from build123d import *

# Parameters (mm, degrees)
F0_W     = 18
F0_H     = 18
F1_DEPTH = 9


with BuildPart() as f1:
    # F0 (on Front) → F1 (new body, symmetric)
    with BuildSketch(Plane.XZ):
        Rectangle(F0_W, F0_H)
    extrude(amount=F1_DEPTH, both=True)


with BuildPart() as f3:
    # F2 (on Front) → F3 (revolve)
    with BuildSketch(Plane.XZ):
        with BuildLine():
            Line((-12.727922, 0), (12.727922, 0))
            ThreePointArc((12.727922, 0), (0, 12.727922), (-12.727922, 0))
        make_face()
    revolve(axis=Axis((0.310661, 0, 0), (1, 0, 0)))


with BuildPart() as f1_1:
    add(f1.part)

    # F4: intersect F3
    add(f3.part, mode=Mode.INTERSECT)


solid = f1_1.part
For this review, take the finished solid that the model builds, in its own axes (mm). Round coordinates to 2 decimals unless told otherwise and drop trailing zeros. Order: outer loops, then holes, each group sorted by start corner. A loop starts at its lowest first (then second) coordinate and runs counter-clockwise, first axis right, second up. Notation, with made-up numbers: (46, -4.5) -> (60, -4.5) arc R20 ccw to (60, 20.5) -> close; hole circle Ø4 at (43.5, -37.75). An arc over 180 degrees is marked (long way). Write item = value, one per line. Start each with the question number.
1) Take a section at B-B on y = 8. State the section outline as (x, z) points, plus the area to 3 significant figures.
2) Take a section at A-A on z = 8.25. State the section outline as (x, y) points.
3) To check wall thickness, follow line 1 (X direction, y = 7.25, z = -6.5); line 2 (X direction, y = -7.75, z = 8.25); line 3 (Z direction, x = 5.25, y = 7.75). State the ranges of each line that lie inside material, in increasing order. Write a range as from..to.
Verdict:
q1.outline = (-9, -4.12) arc R9.9 ccw to (-4.12, -9) -> (4.12, -9) arc R9.9 ccw to (9, -4.12) -> (9, 4.12) arc R9.9 ccw to (4.12, 9) -> (-4.12, 9) arc R9.9 ccw to (-9, 4.12) -> close
q1.area = 288 mm2
q2.outline = (-9, -3.6) arc R9.69 ccw to (-3.6, -9) -> (3.6, -9) arc R9.69 ccw to (9, -3.6) -> (9, 3.6) arc R9.69 ccw to (3.6, 9) -> (-3.6, 9) arc R9.69 ccw to (-9, 3.6) -> close
q3.line_1 = -8.2..8.2
q3.line_2 = -5.82..5.82
q3.line_3 = -8.62..8.62
